from build123d import *

# Parameters (mm, degrees)
F0_R     = 58.136041623
F0_R_2   = 5.7090569563
F1_DEPTH = 127
F2_SIZE  = 5.08
F3_SIZE  = 5.08
F4_D     = 13.2


with BuildPart() as f1:
    # F0 (on Top) → F1 (new body)
    with BuildSketch(Plane.XY):
        Circle(F0_R)
        Circle(F0_R_2, mode=Mode.SUBTRACT)
    extrude(amount=F1_DEPTH)

    # F2
    f2_edges = [f1.edges().sort_by_distance(p)[0] for p in [
        (-58.136042, 0, 127),
        (-5.709057, 0, 127),
    ]]
    chamfer(f2_edges, length=F2_SIZE)

    # F3
    f3_edges = [f1.edges().sort_by_distance(p)[0] for p in [
        (-58.136042, 0, 0),
        (-5.709057, 0, 0),
    ]]
    chamfer(f3_edges, length=F3_SIZE)

    # F4 (through all)
    with Locations(Plane(origin=(0, 0, 0), x_dir=(1, 0, 0), z_dir=(0, 0, -1))):
        with Locations((0, 0)):
            Hole(F4_D / 2)


solid = f1.part
Check sheet for the modelled part. Datum: model origin and axes. Units: mm. Round coordinates to 2 decimals unless told otherwise and drop trailing zeros. Order: outer loops, then holes, each group sorted by start corner. A loop starts at its lowest first (then second) coordinate and runs counter-clockwise, first axis right, second up. Notation, with made-up numbers: M 41,18 L 81,18 A16 cw 81,47 Z; hole C -6,37 d8. An arc over 180 degrees is marked long. One line per item, written item: value. Start each with the question number.
1. Scan lines: line 1 along Y through (x, z) = (0, 55); line 2 along X through (y, z) = (-0.5, 61.5); line 3 along Y through (x, z) = (5, 28). Record each from-to range of solid material in increasing order.
2. Gauge pin test, flat ends, axial feed: P1, Ø8, axis at x = -41, z = 59.5, coming from the +Y side; P2, Ø12, axis at y = -16, z = 69, coming from the -X side; P3, Ø8, axis at y = 34, z = 43, coming from the +X side. Record the tip position at first contact, or that the pin passes through.
3. Section check B-B on z = 85.5. Enter the section's corners in (x, y), and give its area (3 significant figures).
4. Section check A-A on x = 0. Enter the section's corners in (y, z).
5. Release check for a two-part mould opening along Y. For faces 1 (the flat face through (11, 1, 127)), 2 (the cylindrical face through (55.451, 17.462, 62.682)), 3 (the cylindrical face through (4.864, -4.461, 64.33)) record: released by +Y, released by -Y, zero draft, split by the parting line, or undercut.
Results found:
1. line 1: -58.14 to -6.6, 6.6 to 58.14
1. line 2: -58.13 to -6.58, 6.58 to 58.13
1. line 3: -57.92 to -4.31, 4.31 to 57.92
2. P1: y = 44.84
2. P2: x = -57.27
2. P3: x = 49.8
3. outline: C 0,0 d116.27; hole C 0,0 d13.2
3. area: 10,500 mm^2
4. outline: M -58.14,5.08 L -53.06,0 L -10.79,0 L -6.6,4.19 L -6.6,122.81 L -10.79,127 L -53.06,127 L -58.14,121.92 Z; M 6.6,4.19 L 10.79,0 L 53.06,0 L 58.14,5.08 L 58.14,121.92 L 53.06,127 L 10.79,127 L 6.6,122.81 Z
5. face 1: zero draft
5. face 2: split by the parting line
5. face 3: undercut
